from build123d import *

# Parameters (mm, degrees)
BOSS_EXTRUDE1_DEPTH = 40
SKETCH2_R           = 7
CUT_EXTRUDE1_DEPTH  = 25


with BuildPart() as part:
    # Sketch1 → Boss-Extrude1 (new body)
    with BuildSketch(Plane(origin=(0, 0, 0), x_dir=(1, 0, 0), z_dir=(0, 1, 0))):
        Polygon((-46.903241084, -0.468259604), (-46.903241084, -10.468259604), (103.014291308, -15.494982846), (103.014291308, 4.505017154), align=None)
    extrude(amount=BOSS_EXTRUDE1_DEPTH)

    # Sketch2 → Cut-Extrude1 (cut)
    with BuildSketch(Plane(origin=(0, 40, 0), x_dir=(1, 0, 0), z_dir=(0, 1, 0))):
        with Locations((90, -5)):
            Circle(SKETCH2_R)
    extrude(amount=-CUT_EXTRUDE1_DEPTH, mode=Mode.SUBTRACT)


solid = part.part
The listing builds one solid part. Answer for the finished solid, in the listing's coordinates (mm). A direction names the side the tool comes from. Give positions to 0.01 mm unless a question says otherwise; leave off trailing zeros. Write each loop counter-clockwise with the first axis right and the second up, starting at its lowest first coordinate (ties: lowest second). Pieces come first, ordered by that corner, then holes.
1) A tool of negligible diameter and unlimited length cuts with its end or side. For faces 1 (the face through (90, 15, 5)), 2 (the face through (103.014, 20, 6)), from which of +Z, -Z, +X, -X, +Y, -Y can it reach the whole face along a straight path? Write none if from no direction.
2) Section B-B (y = 32.5) is taken. Write down the section's boundary in (x, z).
3) Section A-A (z = 5) is taken. Write down the section's boundary in (x, y), and give its area (3 significant figures).
4) Find the intervals of material crossed by L1, parallel to X at y = 28.25, z = 5; L2, parallel to Y at x = 88.5, z = 8.5; L3, parallel to Z at x = 90, y = 31, in increasing order.
5) Section C-C (x = 90) is taken. Write down the section's boundary in (y, z), and give its area (3 significant figures).
6) For a pull along X with two mould halves and no side action, classify faces 3 (the face through (83, 28, 5)), 4 (the face through (-46.903, 20, 5)), 5 (the face through (44, 0, 5)) as pulls with the +X half, pulls with the -X half, needs draft (parallel to the pull), parting line crosses it, or undercut.
7) Section D-D (x = 73) is taken. Write down the section's boundary in (y, z), and give its area (3 significant figures).
8) Given P1, Ø6, axis at y = 16, z = 11, coming from the -X side; P2, Ø3, axis at x = -31.5, y = 24.5, coming from the -Z side; P3, Ø5, axis at x = 41.5, y = 20.5, coming from the +Z side; P4, Ø7, axis at x = 90, z = 6, coming from the +Y side, each flat-ended and moving along its own axis, determine where each tip first touches the part or whether it passes through.
Response:
1. face 1: +Y
1. face 2: +Z, -Z, +X, +Y, -Y
2. outline: (-46.9, 0.47) - (103.01, -4.51) - (103.01, 15.49) - (-46.9, 10.47) - close; hole circle Ø14 at (90, 5)
3. outline: (-46.9, 0) - (103.01, 0) - (103.01, 40) - (97, 40) - (97, 15) - (83, 15) - (83, 40) - (-46.9, 40) - close
3. area: 5,650 mm2
4. L1: x = -46.9 to 83, 97 to 103.01
4. L2: y = 0 to 15
4. L3: z = -4.07 to -2, 12 to 15.06
5. outline: (0, -4.07) - (40, -4.07) - (40, -2) - (15, -2) - (15, 12) - (40, 12) - (40, 15.06) - (0, 15.06) - close
5. area: 415 mm2
6. face 3: undercut
6. face 4: pulls with the -X half
6. face 5: needs draft
7. outline: (0, -3.51) - (40, -3.51) - (40, 14.49) - (0, 14.49) - close
7. area: 720 mm2
8. P1: stops at x = -46.9
8. P2: stops at z = -0.09
8. P3: stops at z = 13.52
8. P4: stops at y = 15
